Check sheet for the modelled part. Datum: model origin and axes. Units: mm. A direction names the side the tool comes from. Coordinates: 2 decimals unless noted, no trailing zeros. Write each loop counter-clockwise with the first axis right and the second up, starting at its lowest first coordinate (ties: lowest second). Pieces come first, ordered by that corner, then holes. Notation, with made-up numbers: (-21, 34.25) - (-8, 34.25) arc R8 ccw to (-8, 49.25) - close; hole circle Ø3 at (2.25, 47). An arc over 180 degrees is marked (long way). Write each question's results on one line, items separated by ' | '.
from build123d import *

# Parameters (mm, degrees)
F1_DEPTH = 7.1
F2_DEPTH = 25


with BuildPart() as f1:
    # F0 (on Top) → F1 (new body)
    with BuildSketch(Plane.XY):
        with BuildLine():
            Line((-2.752413094, -69.1138580441), (1.247586906, -69.1138580441))
            Line((1.247586906, -69.1138580441), (5.247586906, -69.1138580441))
            ThreePointArc((5.247586906, -69.1138580441), (1.247586906, -65.1138580441), (-2.752413094, -69.1138580441))
        make_face()
        with BuildLine():
            Line((5.247586906, -69.1138580441), (1.247586906, -69.1138580441))
            Line((1.247586906, -69.1138580441), (-2.752413094, -69.1138580441))
            ThreePointArc((-2.752413094, -69.1138580441), (-2.0990532002, -71.3047482742), (-0.352413094, -72.7799186001))
            ThreePointArc((-0.352413094, -72.7799186001), (1.247586906, -73.1138580441), (2.847586906, -72.7799186001))
            ThreePointArc((2.847586906, -72.7799186001), (4.5942270121, -71.3047482742), (5.247586906, -69.1138580441))
        make_face()
        with BuildLine():
            ThreePointArc((-2.752413094, -69.1138580441), (1.247586906, -65.1138580441), (5.247586906, -69.1138580441))
            Line((5.247586906, -69.1138580441), (8.247586906, -69.1138580441))
            ThreePointArc((8.247586906, -69.1138580441), (1.247586906, -62.1138580441), (-5.752413094, -69.1138580441))
            Line((-5.752413094, -69.1138580441), (-2.752413094, -69.1138580441))
        make_face()
        with BuildLine():
            Line((8.247586906, -69.1138580441), (5.247586906, -69.1138580441))
            ThreePointArc((5.247586906, -69.1138580441), (4.5942270121, -71.3047482742), (2.847586906, -72.7799186001))
            Line((2.847586906, -72.7799186001), (8.1125655384, -70.4820935415))
            ThreePointArc((8.1125655384, -70.4820935415), (8.2137497819, -69.8012987954), (8.247586906, -69.1138580441))
        make_face()
        with BuildLine():
            ThreePointArc((-0.352413094, -72.7799186001), (-2.0990532002, -71.3047482742), (-2.752413094, -69.1138580441))
            Line((-2.752413094, -69.1138580441), (-5.752413094, -69.1138580441))
            ThreePointArc((-5.752413094, -69.1138580441), (-5.7185759699, -69.8012987954), (-5.6173917265, -70.4820935415))
            Line((-5.6173917265, -70.4820935415), (-0.352413094, -72.7799186001))
        make_face()
        with BuildLine():
            ThreePointArc((-5.752413094, -69.1138580441), (1.247586906, -62.1138580441), (8.247586906, -69.1138580441))
            Line((8.247586906, -69.1138580441), (11.247586906, -69.1138580441))
            Line((11.247586906, -69.1138580441), (11.247586906, 29.7058020684))
            ThreePointArc((11.247586906, 29.7058020684), (1.247586906, 25.8861419559), (-8.752413094, 29.7058020684))
            Line((-8.752413094, 29.7058020684), (-8.752413094, -69.1138580441))
            Line((-8.752413094, -69.1138580441), (-5.752413094, -69.1138580441))
        make_face()
        with BuildLine():
            Line((11.247586906, -69.1138580441), (8.247586906, -69.1138580441))
            ThreePointArc((8.247586906, -69.1138580441), (8.2137497819, -69.8012987954), (8.1125655384, -70.4820935415))
            Line((8.1125655384, -70.4820935415), (11.247586906, -69.1138580441))
        make_face()
        with BuildLine():
            Line((8.1125655384, -70.4820935415), (2.847586906, -72.7799186001))
            ThreePointArc((2.847586906, -72.7799186001), (1.247586906, -73.1138580441), (-0.352413094, -72.7799186001))
            Line((-0.352413094, -72.7799186001), (-5.6173917265, -70.4820935415))
            ThreePointArc((-5.6173917265, -70.4820935415), (-4.2041963042, -73.5045367877), (-1.552413094, -75.5294640171))
            ThreePointArc((-1.552413094, -75.5294640171), (1.247586906, -76.1138580441), (4.047586906, -75.5294640171))
            ThreePointArc((4.047586906, -75.5294640171), (6.6993701161, -73.5045367877), (8.1125655384, -70.4820935415))
        make_face()
        with BuildLine():
            ThreePointArc((-5.6173917265, -70.4820935415), (-5.7185759699, -69.8012987954), (-5.752413094, -69.1138580441))
            Line((-5.752413094, -69.1138580441), (-8.752413094, -69.1138580441))
            Line((-8.752413094, -69.1138580441), (-5.6173917265, -70.4820935415))
        make_face()
        with BuildLine():
            Line((11.247586906, -72.3871263977), (11.247586906, -69.1138580441))
            Line((11.247586906, -69.1138580441), (8.1125655384, -70.4820935415))
            ThreePointArc((8.1125655384, -70.4820935415), (6.6993701161, -73.5045367877), (4.047586906, -75.5294640171))
            Line((4.047586906, -75.5294640171), (11.247586906, -72.3871263977))
        make_face()
        with BuildLine():
            Line((-5.6173917265, -70.4820935415), (-8.752413094, -69.1138580441))
            Line((-8.752413094, -69.1138580441), (-8.752413094, -72.3871263977))
            Line((-8.752413094, -72.3871263977), (-1.552413094, -75.5294640171))
            ThreePointArc((-1.552413094, -75.5294640171), (-4.2041963042, -73.5045367877), (-5.6173917265, -70.4820935415))
        make_face()
        with BuildLine():
            ThreePointArc((-8.752413094, 29.7058020684), (1.247586906, 25.8861419559), (11.247586906, 29.7058020684))
            Line((11.247586906, 29.7058020684), (11.247586906, 36.1263494184))
            ThreePointArc((11.247586906, 36.1263494184), (1.247586906, 29.8111419559), (-8.752413094, 36.1263494184))
            Line((-8.752413094, 36.1263494184), (-8.752413094, 29.7058020684))
        make_face()
        with BuildLine():
            Line((11.247586906, 36.1263494184), (11.247586906, 29.7058020684))
            ThreePointArc((11.247586906, 29.7058020684), (14.9406508436, 34.7624175989), (16.247586906, 40.8861419559))
            ThreePointArc((16.247586906, 40.8861419559), (-4.876137451, 54.5792058935), (-8.752413094, 29.7058020684))
            Line((-8.752413094, 29.7058020684), (-8.752413094, 36.1263494184))
            ThreePointArc((-8.752413094, 36.1263494184), (-1.1922517158, 51.6890495506), (12.322586906, 40.8861419559))
            ThreePointArc((12.322586906, 40.8861419559), (12.0504945007, 38.4463033341), (11.247586906, 36.1263494184))
        make_face()
    extrude(amount=F1_DEPTH)

    # F0 (on Top) → F2 (join)
    with BuildSketch(Plane.XY):
        with BuildLine():
            Line((-2.752413094, -69.1138580441), (1.247586906, -69.1138580441))
            Line((1.247586906, -69.1138580441), (5.247586906, -69.1138580441))
            ThreePointArc((5.247586906, -69.1138580441), (1.247586906, -65.1138580441), (-2.752413094, -69.1138580441))
        make_face()
        with BuildLine():
            Line((5.247586906, -69.1138580441), (1.247586906, -69.1138580441))
            Line((1.247586906, -69.1138580441), (-2.752413094, -69.1138580441))
            ThreePointArc((-2.752413094, -69.1138580441), (-2.0990532002, -71.3047482742), (-0.352413094, -72.7799186001))
            ThreePointArc((-0.352413094, -72.7799186001), (1.247586906, -73.1138580441), (2.847586906, -72.7799186001))
            ThreePointArc((2.847586906, -72.7799186001), (4.5942270121, -71.3047482742), (5.247586906, -69.1138580441))
        make_face()
    extrude(amount=F2_DEPTH)


solid = f1.part
1. Material ranges on L1, parallel to X at y = -41, z = 5.25; L2, parallel to Z at x = -8.25, y = -69; L3, parallel to Y at x = -5.25, z = 1.75, recorded low to high. Write a range as [from, to].
Values follow:
L1: x = [-8.75, 11.25] | L2: z = [0, 7.1] | L3: y = [-73.92, 31.92], [49.85, 54.41]
2. Sectioned sample at B-B (x = 8.25). Record the cut outline in (y, z).
Values follow:
outline: (-73.7, 0) - (32.31, 0) - (32.31, 7.1) - (-73.7, 7.1) - close; (49.47, 0) - (54.15, 0) - (54.15, 7.1) - (49.47, 7.1) - close
3. Sectioned sample at D-D (y = -56). Record the cut outline in (x, z).
Values follow:
outline: (-8.75, 0) - (11.25, 0) - (11.25, 7.1) - (-8.75, 7.1) - close
4. Go/stop test with flat-tipped pins: pin 1 (5.5 mm diameter, centred on y = -3.5, z = 5.5, fed in from +X); pin 2 (1.5 mm diameter, centred on x = -2.5, y = -24, fed in from +Z); pin 3 (2 mm diameter, centred on x = 4, z = 6, fed in from +Y); pin 4 (5 mm diameter, centred on x = 3, z = 4, fed in from -Y). Record where each tip stops, or that it passes through.
Values follow:
pin 1: stops at x = 11.25 | pin 2: stops at z = 7.1 | pin 3: stops at y = 55.78 | pin 4: stops at y = -76.11
5. Sectioned sample at C-C (z = 23.25). Record the cut outline in (x, y), then the cut area to 3 significant figures.
Values follow:
outline: circle Ø8 at (1.25, -69.11) | area: 50.3 mm^2
6. Access from +Z, -Z, +X, -X, +Y, -Y to the whole of each face (thin tool, end or side, straight path). Record for faces 1 (the flat face through (-5.203, -73.936, 3.5)), 2 (the flat face through (11.248, -22, 4)).
Values follow:
face 1: +Z, -Z, -X, -Y | face 2: +Z, -Z, +X, -Y
7. Sectioned sample at A-A (y = 44). Record the cut outline in (x, z).
Values follow:
outline: (-13.43, 0) - (-9.38, 0) - (-9.38, 7.1) - (-13.43, 7.1) - close; (11.88, 0) - (15.92, 0) - (15.92, 7.1) - (11.88, 7.1) - close
8. Draft check along X on faces 3 (the flat face through (1, -9, 7.1)), 4 (the flat face through (-8.752, -21, 4)), 5 (the cylindrical face through (-1.15, 51.7, 3.5)). Enter one of: pulls with the +X half, pulls with the -X half, needs draft (parallel to the pull), parting line crosses it, or undercut.
Values follow:
face 3: needs draft | face 4: pulls with the -X half | face 5: undercut
